```python
from build123d import *

# Parameters (mm, degrees)
SKETCH1_W               = 84
SKETCH1_H               = 84
BOSS_EXTRUDE1_DEPTH     = 6
SKETCH2_R               = 1.5
CUT_EXTRUDE1_DEPTH      = 119.94536561
SKETCH4_R               = 1.5
CUT_EXTRUDE4_DEPTH      = 3
MIRROR3_COPY_1_SKETCH_R = 1.5
MIRROR3_COPY_1_DEPTH    = 3
SKETCH5_W               = 50
SKETCH5_H               = 32
BOSS_EXTRUDE2_DEPTH     = 22
SKETCH6_W               = 44
SKETCH6_H               = 26
CUT_EXTRUDE5_DEPTH      = 25
SKETCH8_R               = 5.5
CUT_EXTRUDE14_DEPTH     = 22
CUT_EXTRUDE15_DEPTH     = 122.396046064
FILLET2_R               = 5
FILLET3_R               = 5


with BuildPart() as part:
    # Sketch1 → Boss-Extrude1 (new body)
    with BuildSketch(Plane(origin=(0, 0, 0), x_dir=(1, 0, 0), z_dir=(0, 1, 0))):
        with Locations((42, 42)):
            Rectangle(SKETCH1_W, SKETCH1_H)
    extrude(amount=BOSS_EXTRUDE1_DEPTH)

    # Sketch2 → Cut-Extrude1 (cut, through all)
    with BuildSketch(Plane(origin=(0, 6, 0), x_dir=(1, 0, 0), z_dir=(0, 1, 0))):
        with Locations(Location((6, 72, 0), (0, 0, 270))):
            Circle(SKETCH2_R)
        with Locations(Location((6, 12, 0), (0, 0, 270))):
            Circle(SKETCH2_R)
        with Locations(Location((78, 12, 0), (0, 0, 270))):
            Circle(SKETCH2_R)
        with Locations(Location((78, 72, 0), (0, 0, 270))):
            Circle(SKETCH2_R)
    extrude(amount=-CUT_EXTRUDE1_DEPTH, mode=Mode.SUBTRACT)

    # Sketch4 → Cut-Extrude4 (cut)
    with BuildSketch(Plane(origin=(0, 6, 0), x_dir=(1, 0, 0), z_dir=(0, 1, 0))):
        Polygon((13, 15), (13, 9), (3, 9), (3, 21), (8, 21), align=None)
        with Locations(Location((6, 12, 0), (0, 0, 270))):
            Circle(SKETCH4_R, mode=Mode.SUBTRACT)
    cut_extrude4 = extrude(amount=-CUT_EXTRUDE4_DEPTH, mode=Mode.SUBTRACT)

    # Mirror2: Cut-Extrude4 across plane
    add(cut_extrude4.mirror(Plane.XY.offset(-42)), mode=Mode.SUBTRACT)

    # Mirror3: Cut-Extrude4 across plane
    add(cut_extrude4.mirror(Plane.ZY.offset(-42)), mode=Mode.SUBTRACT)

    # Mirror3 copy 1 sketch → Mirror3 copy 1 (cut)
    with BuildSketch(Plane(origin=(84, 6, -84), x_dir=(-1, 0, 0), z_dir=(0, 1, 0))):
        Polygon((13, 15), (13, 9), (3, 9), (3, 21), (8, 21), align=None)
        with Locations(Location((6, 12, 0), (0, 0, 270))):
            Circle(MIRROR3_COPY_1_SKETCH_R, mode=Mode.SUBTRACT)
    extrude(amount=-MIRROR3_COPY_1_DEPTH, mode=Mode.SUBTRACT)

    # Sketch5 → Boss-Extrude2 (add)
    with BuildSketch(Plane(origin=(0, 6, 0), x_dir=(1, 0, 0), z_dir=(0, 1, 0))):
        with Locations((50, 16)):
            Rectangle(SKETCH5_W, SKETCH5_H)
    extrude(amount=BOSS_EXTRUDE2_DEPTH)

    # Sketch6 → Cut-Extrude5 (cut)
    with BuildSketch(Plane(origin=(0, 28, 0), x_dir=(1, 0, 0), z_dir=(0, 1, 0))):
        with Locations((50, 16)):
            Rectangle(SKETCH6_W, SKETCH6_H)
    extrude(amount=-CUT_EXTRUDE5_DEPTH, mode=Mode.SUBTRACT)

    # Sketch8 → Cut-Extrude14 (cut)
    with BuildSketch(Plane(origin=(0, 28, 0), x_dir=(1, 0, 0), z_dir=(0, 1, 0))):
        with Locations((78, 12)):
            Circle(SKETCH8_R)
    extrude(amount=-CUT_EXTRUDE14_DEPTH, mode=Mode.SUBTRACT)

    # Sketch13 → Cut-Extrude15 (cut, through all)
    with BuildSketch(Plane(origin=(0, 3, 0), x_dir=(1, 0, 0), z_dir=(0, 1, 0))):
        Polygon((72, 9), (81, 9), (81, 21), (76, 21), (72, 16.2), (72, 29), (28, 29), (28, 3), (72, 3), align=None)
    extrude(amount=CUT_EXTRUDE15_DEPTH, mode=Mode.SUBTRACT)

    # Fillet2
    fillet2_edges = [part.edges().sort_by_distance(p)[0] for p in [
        (75, 17, -32),
        (25, 17, -32),
    ]]
    fillet(fillet2_edges, radius=FILLET2_R)

    # Fillet3
    fillet3_edges = [part.edges().sort_by_distance(p)[0] for p in [
        (72, 15.5, -29),
        (72, 3, -6),
        (50, 3, -3),
        (72, 15.5, -3),
        (28, 3, -16),
        (28, 15.5, -3),
        (50, 3, -29),
        (28, 15.5, -29),
    ]]
    fillet(fillet3_edges, radius=FILLET3_R)


solid = part.part
```
Input: part model. Units: mm. Frame: model coordinates. A direction names the side the tool comes from. Give positions to 0.01 mm unless a question says otherwise; leave off trailing zeros. Loops run counter-clockwise (first coordinate to the right, second up) from the corner with the lowest first, then second, coordinate; pieces in that order, holes last.
1) Contact query for flat-ended pins moving along their axis: pin 1 (2.5 mm diameter, centred on y = 4.5, z = -68.5, fed in from -X); pin 2 (8.5 mm diameter, centred on y = 14, z = -22, fed in from -X); pin 3 (8 mm diameter, centred on y = 15.5, z = -4.5, fed in from +X); pin 4 (15.5 mm diameter, centred on x = 76.5, y = 14, fed in from -Z). Output: stop coordinate, or through.
A:
pin 1: stops at x = 0
pin 2: stops at x = 25
pin 3: stops at x = 75
pin 4: stops at z = -32
2) Mould query, pull axis Z, two halves, no side actions, for faces 1 (the flat face through (84, 3, -41)), 2 (the flat face through (8, 5, -9)), 3 (the cylindrical face through (26, 17, -30)). Classes: released by +Z, released by -Z, zero draft, split by the parting line, or undercut.
A:
face 1: zero draft
face 2: undercut
face 3: released by -Z
3) Reachability of faces 4 (the flat face through (75, 17, -4)), 5 (the flat face through (73.584, 15.675, -18.1)), 6 (the cylindrical face through (74, 17, -30)) from +Z, -Z, +X, -X, +Y, -Y: full face, straight path, thin tool, end or side. Return the list, or none.
A:
face 4: +Z, -Z, +X, +Y
face 5: +Y
face 6: -Z, +X, +Y
4) Section query B-B on x = 6. Return the cut outline in (y, z), and give its area (3 significant figures).
A:
outline: (0, -84) - (6, -84) - (6, -75) - (3, -75) - (3, -73.5) - (0, -73.5) - close; (0, -70.5) - (3, -70.5) - (3, -63) - (6, -63) - (6, -21) - (3, -21) - (3, -13.5) - (0, -13.5) - close; (0, -10.5) - (3, -10.5) - (3, -9) - (6, -9) - (6, 0) - (0, 0) - close
area: 414 mm2
5) Line query: L1, parallel to X at y = 2.2, z = -72; L2, parallel to Z at x = 78, y = 2.2; L3, parallel to Z at x = 39.5, y = 11. Output: solid intervals per line, ascending.
A:
L1: x = 0 to 4.5, 7.5 to 76.5, 79.5 to 84
L2: z = -84 to -73.5, -70.5 to -13.5, -10.5 to 0
L3: z = -32 to -29, -3 to 0
6) Section query A-A on z = -12. Return the cut outline in (x, y).
A:
outline: (0, 0) - (4.5, 0) - (4.5, 3) - (3, 3) - (3, 6) - (0, 6) - close; (7.5, 0) - (76.5, 0) - (76.5, 3) - (33, 3) arc R5 cw to (28, 8) - (28, 28) - (25, 28) - (25, 6) - (13, 6) - (13, 3) - (7.5, 3) - close; (79.5, 0) - (84, 0) - (84, 6) - (81, 6) - (81, 3) - (79.5, 3) - close
7) Section query D-D on x = 61. Return the cut outline in (y, z), and give its area (3 significant figures).
A:
outline: (0, -84) - (6, -84) - (6, -32) - (28, -32) - (28, -29) - (8, -29) arc R5 cw to (3, -24) - (3, -8) arc R5 cw to (8, -3) - (28, -3) - (28, 0) - (0, 0) - close
area: 569 mm2
8) Section query C-C on y = 23.75. Return the cut outline in (x, z), and give its area (3 significant figures).
A:
outline: (25, -27) arc R5 ccw to (30, -32) - (70, -32) arc R5 ccw to (75, -27) - (75, -19.8) - (72, -16.2) - (72, -24) arc R5 cw to (67, -29) - (33, -29) arc R5 cw to (28, -24) - (28, -8) arc R5 cw to (33, -3) - (67, -3) arc R5 cw to (72, -8) - (72, -9) - (73.39, -9) arc R5.5 cw to (75, -7.39) - (75, 0) - (25, 0) - close
area: 438 mm2
